The figure shows three views and two pictorial views of one solid part (mm, origin at its lowest corner). Answer the questions. Coordinates: 2 decimals unless noted, no trailing zeros. Loops run counter-clockwise (first coordinate to the right, second up) from the corner with the lowest first, then second, coordinate; pieces in that order, holes last. Notation, with made-up numbers: M 10,83.5 L 38,83.5 A17 ccw 38,102.5 Z; hole C 8,-20 d9. An arc over 180 degrees is marked long. Return JSON: item names as keys, results as strings. Group by question number.
1. Given P1, Ø8, axis at x = 64.5, y = 78, coming from the +Z side; P2, Ø2.5, axis at x = 8, z = 5.5, coming from the -Y side; P3, Ø2.5, axis at y = 4, z = 4, coming from the +X side; P4, Ø2.5, axis at y = 4, z = 3, coming from the -X side, each flat-ended and moving along its own axis, determine where each tip first touches the part or whether it passes through.
2. Section A-A (z = 4.25) is taken. Write down the section's boundary in (x, y).
3. The mould has two halves that part along Y. Classify the marked faces 1 and 2: pulls with the +Y half, pulls with the -Y half, needs draft (parallel to the pull), parting line crosses it, or undercut.
4. Straight lines are drawn through the part: L1, parallel to Y at x = 85, z = 6.5; L2, parallel to Z at x = 59, y = 96. For each, find the intervals that lie inside material, in ascending order. Write a range as from..to.
5. Section B-B (x = 62.5) is taken. Write down the section's boundary in (y, z).
6. Section D-D (x = 102) is taken. Write down the section's boundary in (y, z).
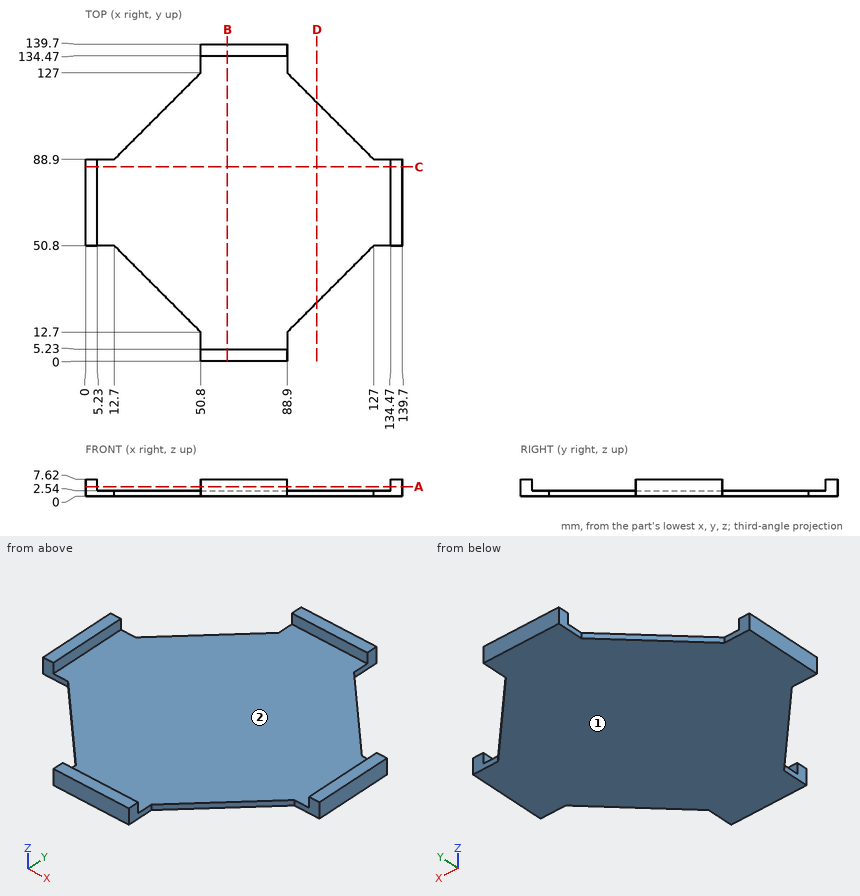
Worked out:
{
 "1": {"P1": "z = 2.54", "P2": "through", "P3": "x = 88.9", "P4": "x = 50.8"},
 "2": {"outline": "M 0,50.8 L 5.23,50.8 L 5.23,88.9 L 0,88.9 Z; M 50.8,0 L 88.9,0 L 88.9,5.23 L 50.8,5.23 Z; M 50.8,134.47 L 88.9,134.47 L 88.9,139.7 L 50.8,139.7 Z; M 134.47,50.8 L 139.7,50.8 L 139.7,88.9 L 134.47,88.9 Z"},
 "3": {"face 1": "needs draft", "face 2": "undercut"},
 "4": {"L1": "0..5.23, 134.47..139.7", "L2": "0..2.54"},
 "5": {"outline": "M 0,0 L 139.7,0 L 139.7,7.62 L 134.47,7.62 L 134.47,2.54 L 5.23,2.54 L 5.23,7.62 L 0,7.62 Z"},
 "6": {"outline": "M 25.8,0 L 113.9,0 L 113.9,2.54 L 25.8,2.54 Z"}
}
